```python
from build123d import *

# Parameters (mm, degrees)
PROFILE_EXTRUDE_DEPTH               = 34
GUSSET_1_EXTRUDE_DEPTH              = 3
GUSSET_START                        = 31
GUSSET_2_EXTRUDE_DEPTH              = 3
SOLENOID_MOUNTING_HOLES_D           = 3.4
SOLENOID_MOUNTING_HOLES_CBORE_D     = 7
SOLENOID_MOUNTING_HOLES_CBORE_DEPTH = 3.9
M3_MOUNTING_HOLES_D                 = 3.4
FRONT_START                         = -1
FRONT_EDGE_FILLETS_DEPTH            = 36
FRONT_EDGE_FILLETS_2_DEPTH          = 34
TOP_START                           = -1
TOP_EDGE_FILLET_DEPTH               = 36
CORNER_FILLETS_R                    = 1.5


with BuildPart() as part:
    # Profile Sketch → Profile  Extrude (new body)
    with BuildSketch(Plane.XY):
        Polygon((0, 0), (0, 3.5), (-20, 3.5), (-20, -3), (12, -3), (12, 0), align=None)
    extrude(amount=PROFILE_EXTRUDE_DEPTH)

    # Gusset Sketch → Gusset 1 Extrude (add)
    with BuildSketch(Plane.XY):
        Polygon((0, 0), (12, 0), (0, 3.5), align=None)
    extrude(amount=GUSSET_1_EXTRUDE_DEPTH)

    # Gusset Sketch<2> → Gusset 2 Extrude (add)
    with BuildSketch(Plane.XY.offset(GUSSET_START)):
        Polygon((0, 0), (12, 0), (0, 3.5), align=None)
    extrude(amount=GUSSET_2_EXTRUDE_DEPTH)

    # Solenoid Mounting Holes (through all)
    with Locations(Plane(origin=(-3, -3, 0), x_dir=(0, 0, -1), z_dir=(0, -1, 0))):
        with Locations((-9.5, -12), (-24.5, -12), (-24.5, -2), (-9.5, -2)):
            CounterBoreHole(SOLENOID_MOUNTING_HOLES_D / 2, SOLENOID_MOUNTING_HOLES_CBORE_D / 2, SOLENOID_MOUNTING_HOLES_CBORE_DEPTH)

    # M3 Mounting Holes (through all)
    with Locations(Plane(origin=(0, 0, 0), x_dir=(1, 0, 0), z_dir=(0, 1, 0))):
        with Locations((6, -24.5), (6, -9.5)):
            Hole(M3_MOUNTING_HOLES_D / 2)

    # Front Edge Fillets: read off the stored shape, not the designer's step
    # Front Edge Fillets outline → Front Edge Fillets (cut)
    with BuildSketch(Plane.XY.offset(FRONT_START)):
        with BuildLine():
            Line((12, -1.125), (12, 0))
            Line((12, 0), (10.92, 0.315))
            ThreePointArc((10.92, 0.315), (11.7, -0.225), (12, -1.125))
        make_face()
    extrude(amount=FRONT_EDGE_FILLETS_DEPTH, mode=Mode.SUBTRACT)

    # Front Edge Fillets 2 outline → Front Edge Fillets 2 (add)
    with BuildSketch(Plane.XY):
        with BuildLine():
            ThreePointArc((1.5, 0), (0.439339828, 0.439339828), (0, 1.5))
            Line((0, 1.5), (0, 0))
            Line((0, 0), (1.5, 0))
        make_face()
    extrude(amount=FRONT_EDGE_FILLETS_2_DEPTH)

    # Top Edge Fillet: read off the stored shape, not the designer's step
    # Top Edge Fillet outline → Top Edge Fillet (cut)
    with BuildSketch(Plane.XY.offset(TOP_START)):
        with BuildLine():
            Line((1.371428571, 3.1), (0, 3.5))
            Line((0, 3.5), (-1.428571429, 3.5))
            ThreePointArc((-1.428571429, 3.5), (-0.014357867, 3.399494937), (1.371428571, 3.1))
        make_face()
    extrude(amount=TOP_EDGE_FILLET_DEPTH, mode=Mode.SUBTRACT)

    # Corner Fillets
    corner_fillets_edges = [part.edges().sort_by_distance(p)[0] for p in [
        (-10.714285714, 3.5, 0),
        (-10.714285714, 3.5, 34),
        (-0.014357867, 3.399494937, 0),
        (-0.014357867, 3.399494937, 34),
        (-20, 3.5, 17),
        (-20, 0.25, 34),
        (12, -2.0625, 34),
        (12, -2.0625, 0),
        (-20, 0.25, 0),
        (6.145714286, 1.7075, 0),
        (11.7, -0.225, 0),
        (6.145714286, 1.7075, 34),
        (11.7, -0.225, 34),
    ]]
    fillet(corner_fillets_edges, radius=CORNER_FILLETS_R)


solid = part.part
```
The model under review builds one solid part; all positions refer to its coordinate system, in mm. A direction names the side the tool comes from. Give positions to 0.01 mm unless a question says otherwise; leave off trailing zeros. Write each loop counter-clockwise with the first axis right and the second up, starting at its lowest first coordinate (ties: lowest second). Pieces come first, ordered by that corner, then holes. Notation, with made-up numbers: (-28, 19) -> (3, 19) arc R23 cw to (3, 41) -> close; hole circle Ø1 at (-11.5, 32.5). An arc over 180 degrees is marked (long way). Put each result on its own line as item: value.
(1) We need section A-A, the plane x = -15. Give the boundary of the cut face in (y, z), and give its area (3 significant figures).
Results are:
outline: (-3, 0) -> (2, 0) arc R1.5 ccw to (3.5, 1.5) -> (3.5, 7.8) -> (0.9, 7.8) -> (0.9, 6) -> (-3, 6) -> close; (-3, 13) -> (0.9, 13) -> (0.9, 11.2) -> (3.5, 11.2) -> (3.5, 22.8) -> (0.9, 22.8) -> (0.9, 21) -> (-3, 21) -> close; (-3, 28) -> (0.9, 28) -> (0.9, 26.2) -> (3.5, 26.2) -> (3.5, 32.5) arc R1.5 ccw to (2, 34) -> (-3, 34) -> close
area: 148 mm²
(2) We need section D-D, the plane z = 30. Give the boundary of the cut face in (x, y) (3 decimals).
Results are:
outline: (-20, -3) -> (12, -3) -> (12, -1.125) arc R1.5 ccw to (11.492, 0) -> (1.5, 0) arc R1.5 cw to (0, 1.5) -> (0, 3.397) arc R10 ccw to (-1.429, 3.5) -> (-18.5, 3.5) arc R1.5 ccw to (-20, 2) -> close
(3) Tool access review of faces 1 (the cylindrical face through (-18.105, -1.077, 22.885)), 2 (the flat face through (-4, -3, 17)): name each direction out of +Z, -Z, +X, -X, +Y, -Y from which nothing blocks a thin tool from reaching the whole face with its end or side.
Results are:
face 1: -Y
face 2: +Z, -Z, +X, -X, -Y
(4) We need section B-B, the plane y = -1.75. Give the boundary of the cut face in (x, z), and give its area (3 significant figures).
Results are:
outline: (-20, 1.5) arc R1.5 ccw to (-18.5, 0) -> (10.5, 0) arc R1.5 ccw to (12, 1.5) -> (12, 32.5) arc R1.5 ccw to (10.5, 34) -> (-18.5, 34) arc R1.5 ccw to (-20, 32.5) -> close; hole circle Ø7 at (-15, 9.5); hole circle Ø7 at (-15, 24.5); hole circle Ø7 at (-5, 9.5); hole circle Ø7 at (-5, 24.5); hole circle Ø3.4 at (6, 9.5); hole circle Ø3.4 at (6, 24.5)
area: 914 mm²
(5) The part is to be moulded in two halves that separate along Z. For faces 3 (the flat face through (-7, 0.9, 10)), 4 (the cylindrical face through (-19.55, -0.54, 0.43)), 5 (the flat face through (6.21, 1.69, 2.24)), say which applies: pulls with the +Z half, pulls with the -Z half, needs draft (parallel to the pull), parting line crosses it, or undercut.
Results are:
face 3: undercut
face 4: pulls with the -Z half
face 5: needs draft
(6) We need section C-C, the plane z = 9.5. State how many separate pieces and enclosed holes the cut face has, and give its area (3 significant figures).
Results are:
separate pieces: 4
enclosed holes: 0
area: 83.3 mm²
(7) For pin 1 Ø2 at (x, z) = (-5.5, 8) entering from -Y; pin 2 Ø2.5 at (x, z) = (-15, 9.5) entering from -Y; pin 3 Ø2 at (y, z) = (2.5, 22) entering from +X, all flat-tipped, find the tip position at first contact; note any pin that passes through.
Results are:
pin 1: y = 0.9
pin 2: through
pin 3: x = 0
(8) To check wall thickness, follow probe 1 along X at (y, z) = (-1.8, 24.5); probe 2 along Z at (x, y) = (6, -1.5); probe 3 along Z at (x, y) = (-16, 3). State the ranges of each line that lie inside material, in increasing order. Write a range as from..to.
Results are:
probe 1: -20..-18.5, -11.5..-8.5, -1.5..4.3, 7.7..12
probe 2: 0..7.8, 11.2..22.8, 26.2..34
probe 3: 0.38..8.13, 10.87..23.13, 25.87..33.62
